The drawing under review shows one solid part. Ordinate dimensions are in mm from its lowest x, y, z. A direction names the side the tool comes from. Round coordinates to 2 decimals unless told otherwise and drop trailing zeros. Write each loop counter-clockwise with the first axis right and the second up, starting at its lowest first coordinate (ties: lowest second). Pieces come first, ordered by that corner, then holes. Notation, with made-up numbers: M -12,-4 L 35,-4 A25 cw 35,32 Z; hole C -37.75,24.25 d11. An arc over 180 degrees is marked long. Write item = value, one per line. Start each with the question number.
Item 1: Take a section at A-A, the plane z = 32. Give the boundary of the cut face in (x, y), plus the area to 3 significant figures.
Item 2: Take a section at C-C, the plane x = 19.25. Give the boundary of the cut face in (y, z).
Item 3: Tool access review of the marked faces 1, 2, 3 and 4: name each direction out of +Z, -Z, +X, -X, +Y, -Y from which nothing blocks a thin tool from reaching the whole face with its end or side.
Item 4: Take a section at B-B, the plane y = 32. Give the boundary of the cut face in (x, z), plus the area to 3 significant figures.
Item 5: To check wall thickness, follow line 1 along Y through (x, z) = (20.75, 17); line 2 along X through (y, z) = (30.5, 32). State the ranges of each line that lie inside material, in increasing order.
Item 6: For pin 1 Ø5 at (x, z) = (21, 56.5) entering from -Y; pin 2 Ø4 at (x, y) = (19, 51.5) entering from +Z; pin 3 Ø11 at (x, z) = (18.5, 18) entering from +Y, all flat-tipped, find the tip position at first contact; note any pin that passes through.
Item 7: The part is to be moulded in two halves that separate along Y. For the marked faces 5, 6, 7 and 8, say which applies: +Y half, -Y half, draft (parallel to the pull), parting line (faces both ways), or undercut.
Item 8: Take a section at D-D, the plane y = 59. Give the boundary of the cut face in (x, z).
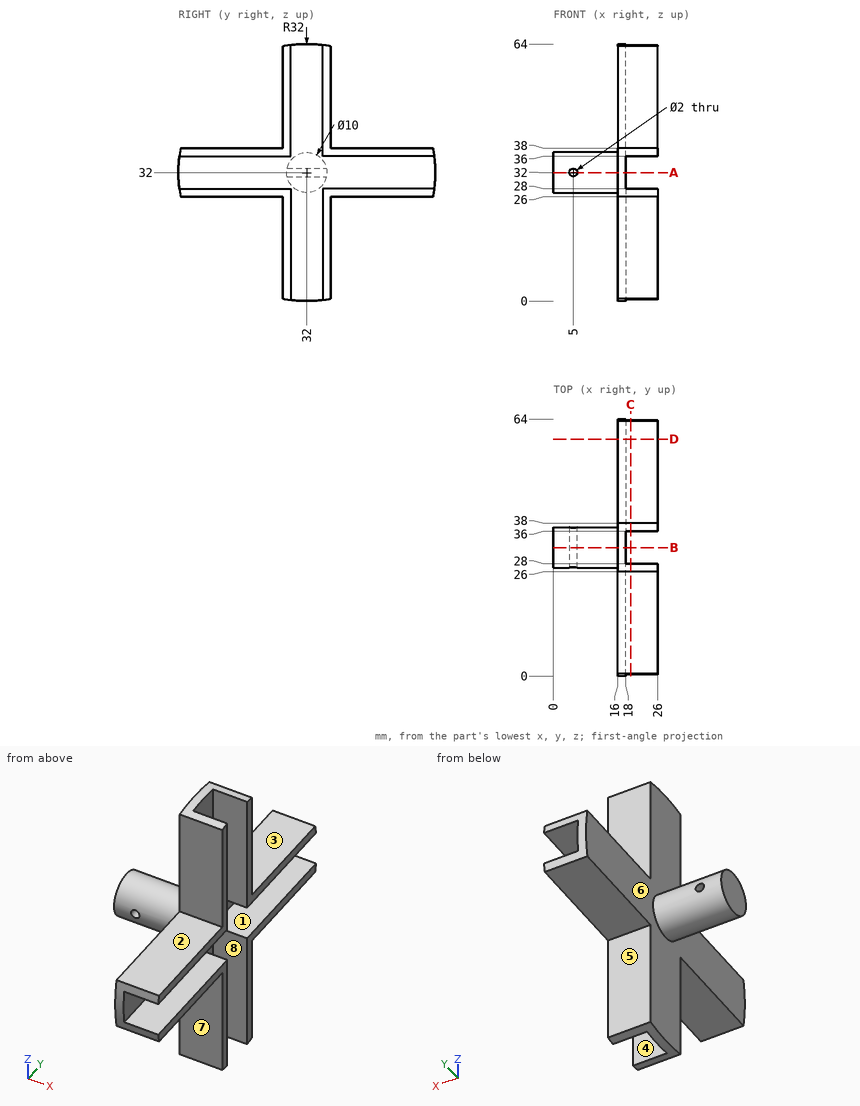
Response values:
q1.outline = M 0,27 L 4,27 L 4,37 L 0,37 Z; M 6,27 L 16,27 L 16,0 L 18,0 L 18,64 L 16,64 L 16,37 L 6,37 Z
q1.area = 268 mm2
q2.outline = M 0.25,28 A32 ccw 0.57,26 L 26,26 L 26,0.57 A32 ccw 28,0.25 L 28,28 Z; M 0.25,36 L 28,36 L 28,63.75 A32 ccw 26,63.43 L 26,38 L 0.57,38 A32 ccw Z; M 36,0.25 A32 ccw 38,0.57 L 38,26 L 63.43,26 A32 ccw 63.75,28 L 36,28 Z; M 36,36 L 63.75,36 A32 ccw 63.43,38 L 38,38 L 38,63.43 A32 ccw 36,63.75 Z
q3.face_1 = +X, +Y, -Y
q3.face_2 = +Z, +X, -X, -Y
q3.face_3 = +Z, +X, -X, +Y
q3.face_4 = +Z, -Z, +X
q4.outline = M 0,27 L 16,27 L 16,0 L 18,0 L 18,64 L 16,64 L 16,37 L 0,37 Z; hole C 5,32 d2
q4.area = 285 mm2
q5.line_1 = 26 to 28, 36 to 38
q5.line_2 = 0 to 4, 6 to 18
q6.pin_1 = 26
q6.pin_2 = 38
q6.pin_3 = 38
q7.face_5 = +Y half
q7.face_6 = draft
q7.face_7 = -Y half
q7.face_8 = undercut
q8.outline = M 16,26 L 26,26 L 26,28 L 18,28 L 18,36 L 26,36 L 26,38 L 16,38 Z
